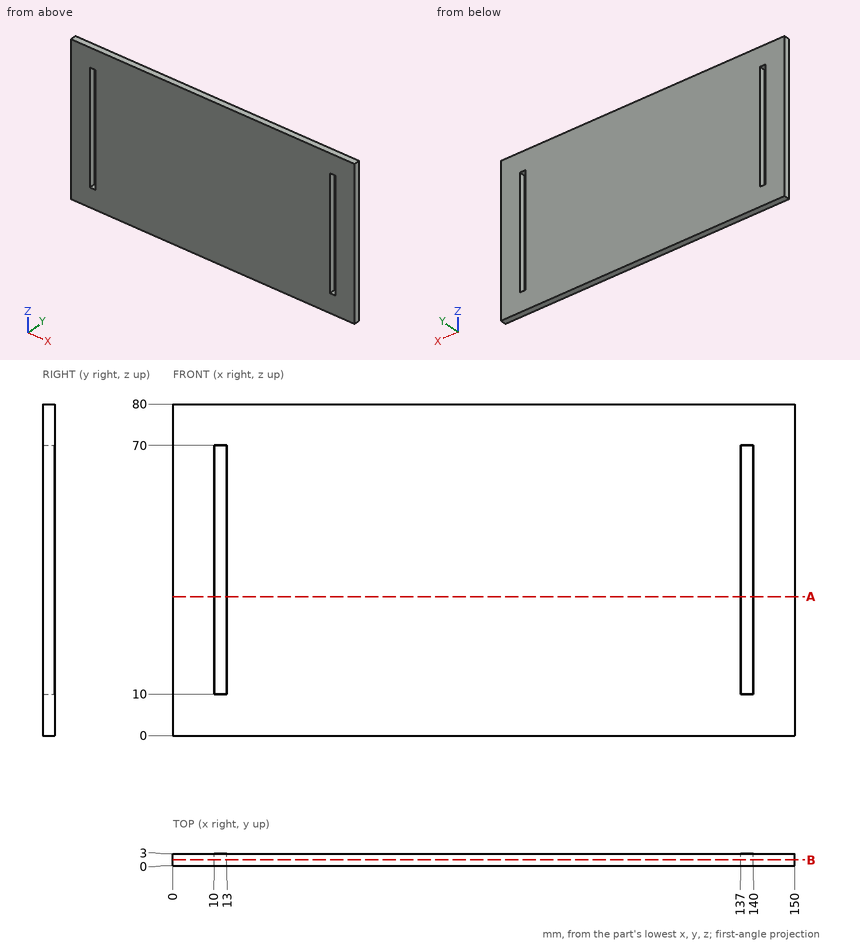
Verification items for this drawing (mm, ordinates from the low corner). Give positions to 0.01 mm unless a question says otherwise; leave off trailing zeros. Loops run counter-clockwise (first coordinate to the right, second up) from the corner with the lowest first, then second, coordinate; pieces in that order, holes last. Notation, with made-up numbers: M -32,16.5 L -7,16.5 A13 cw -7,38.5 Z; hole C 83.5,-14.75 d7. An arc over 180 degrees is marked long. Answer as a JSON object with one key per item and string values. Group by question number.
Item 1: Sectioned sample at A-A on z = 33.5. Record the boundary of the cut face in (x, y), plus the area to 3 significant figures.
Item 2: Material ranges on L1, parallel to X at y = 2.25, z = 47.5; L2, parallel to Z at x = 11.5, y = 1.1, recorded low to high.
Item 3: Sectioned sample at B-B on y = 1.45. Record the boundary of the cut face in (x, z), plus the area to 3 significant figures.
Findings below:
{
 "1": {"outline": "M 0,0 L 10,0 L 10,3 L 0,3 Z; M 13,0 L 137,0 L 137,3 L 13,3 Z; M 140,0 L 150,0 L 150,3 L 140,3 Z", "area": "432 mm2"},
 "2": {"L1": "0 to 10, 13 to 137, 140 to 150", "L2": "0 to 10, 70 to 80"},
 "3": {"outline": "M 0,0 L 150,0 L 150,80 L 0,80 Z; hole M 10,10 L 13,10 L 13,70 L 10,70 Z; hole M 137,10 L 140,10 L 140,70 L 137,70 Z", "area": "11,600 mm2"}
}
